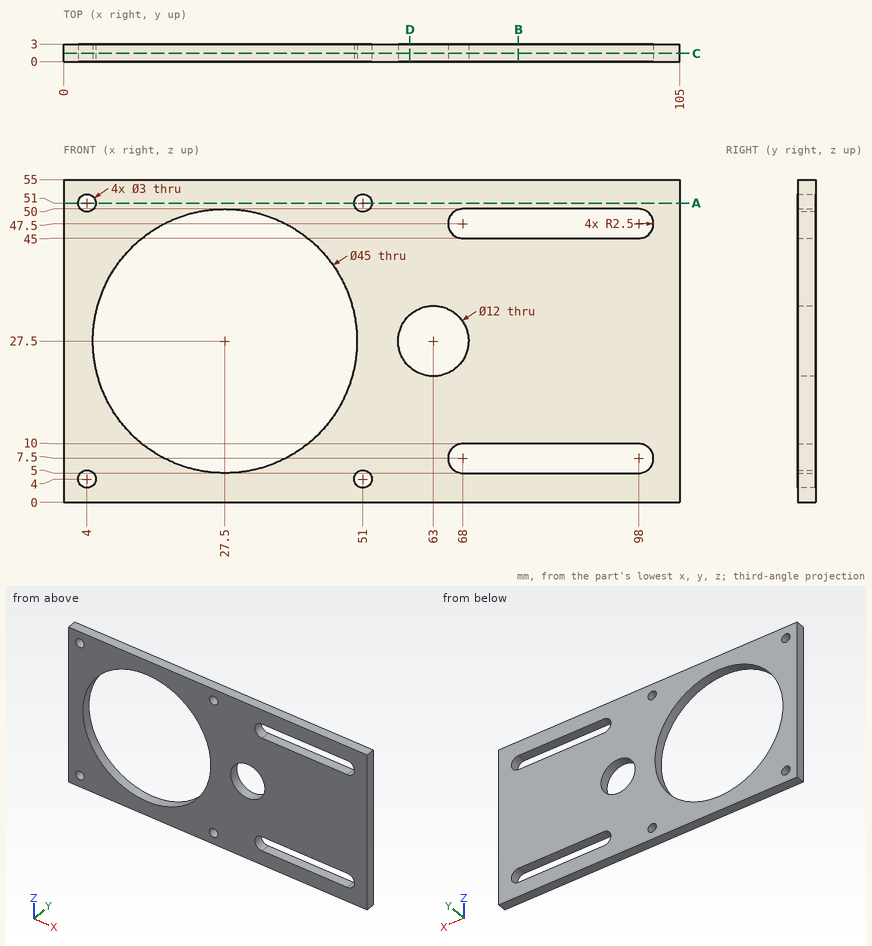
Job drawing, mm, ordinate dimensions from the low corner. One solid piece. Coordinates: 2 decimals unless noted, no trailing zeros. Write each loop counter-clockwise with the first axis right and the second up, starting at its lowest first coordinate (ties: lowest second). Pieces come first, ordered by that corner, then holes. Notation, with made-up numbers: M -34,2 L 21,2 A14 cw 21,15 Z; hole C 38.25,-10 d10. An arc over 180 degrees is marked long. Answer as a JSON object with one key per item and string values. Group by question number.
1) Saw through at A-A (z = 51). Write the cut outline in (x, y).
2) Saw through at D-D (x = 59). Write the cut outline in (y, z).
3) Saw through at B-B (x = 77.5). Write the cut outline in (y, z).
4) Wall check: line 1 (X direction, y = 2.2, z = 27.5); line 2 (X direction, y = 2.3, z = 4); line 3 (Z direction, x = 94, y = 2.2). Give the ranges that are in metal, low to high. Write a range as from..to.
5) Saw through at C-C (y = 1.4). Give the number of separate pieces and of enclosed holes in the cut face, plus the area to 3 significant figures.
6) Pin check, flat tip, straight feed: pin 1 Ø1.8 at (x, z) = (4, 4) entering from -Y. Stop position of the tip, or through.
Values follow:
{
 "1": {"outline": "M 0,0 L 2.5,0 L 2.5,3 L 0,3 Z; M 5.5,0 L 49.5,0 L 49.5,3 L 5.5,3 Z; M 52.5,0 L 105,0 L 105,3 L 52.5,3 Z"},
 "2": {"outline": "M 0,0 L 3,0 L 3,23.03 L 0,23.03 Z; M 0,31.97 L 3,31.97 L 3,55 L 0,55 Z"},
 "3": {"outline": "M 0,0 L 3,0 L 3,5 L 0,5 Z; M 0,10 L 3,10 L 3,45 L 0,45 Z; M 0,50 L 3,50 L 3,55 L 0,55 Z"},
 "4": {"line 1": "x = 0..5, 50..57, 69..105", "line 2": "x = 0..2.5, 5.5..49.5, 52.5..105", "line 3": "z = 0..5, 10..45, 50..55"},
 "5": {"separate pieces": "1", "enclosed holes": "8", "area": "3,700 mm2"},
 "6": {"pin 1": "passes through"}
}
